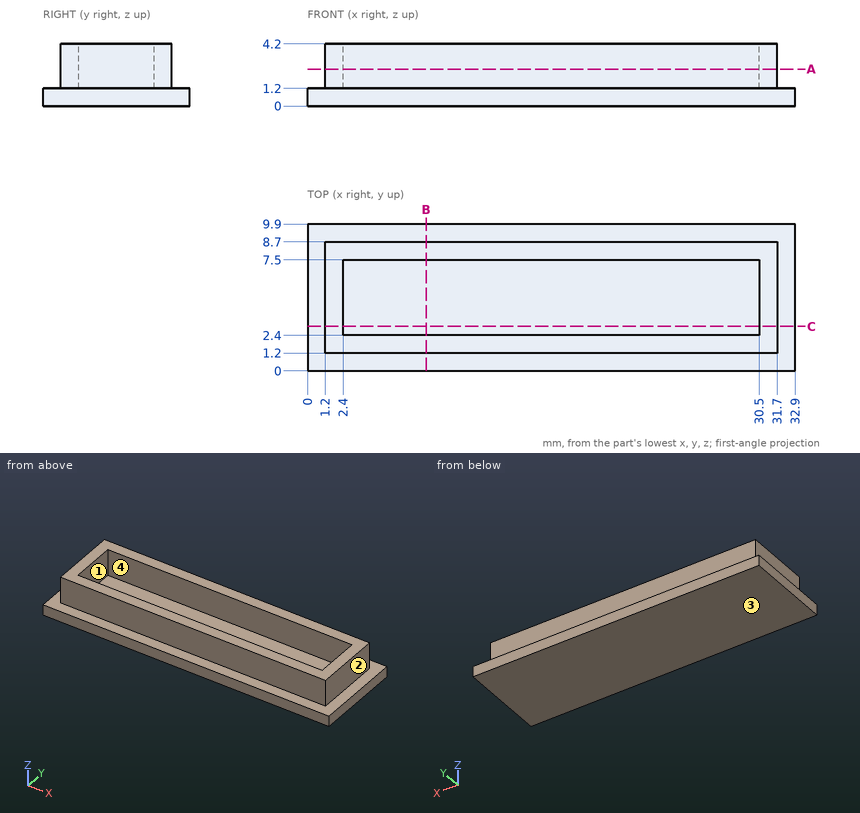
Geometry check sheet. Reference: drawing and pictorial views, mm from the part's lowest x, y, z. Coordinates: 2 decimals unless noted, no trailing zeros. Write each loop counter-clockwise with the first axis right and the second up, starting at its lowest first coordinate (ties: lowest second). Pieces come first, ordered by that corner, then holes.
Item 1: Cross-section at A-A on z = 2.5. Record the boundary of the cut face in (x, y).
Numbers:
outline: (1.2, 1.2) - (31.7, 1.2) - (31.7, 8.7) - (1.2, 8.7) - close; hole (2.4, 2.4) - (30.5, 2.4) - (30.5, 7.5) - (2.4, 7.5) - close
Item 2: Cross-section at C-C on y = 3. Record the boundary of the cut face in (x, z), then the cut area to 3 significant figures.
Numbers:
outline: (0, 0) - (32.9, 0) - (32.9, 1.2) - (31.7, 1.2) - (31.7, 4.2) - (30.5, 4.2) - (30.5, 1.2) - (2.4, 1.2) - (2.4, 4.2) - (1.2, 4.2) - (1.2, 1.2) - (0, 1.2) - close
area: 46.7 mm2
Item 3: Depth check by flat-ended pin: pin 1 Ø2.5 at (x, z) = (14.5, 3) entering from +Y; pin 2 Ø2.5 at (x, y) = (19, 6) entering from +Z; pin 3 Ø0.9 at (y, z) = (4, 3.5) entering from -X. Enter the tip coordinate at first touch or a pass-through.
Numbers:
pin 1: stops at y = 8.7
pin 2: stops at z = 1.2
pin 3: stops at x = 1.2
Item 4: Cross-section at B-B on x = 8. Record the boundary of the cut face in (y, z), then the cut area to 3 significant figures.
Numbers:
outline: (0, 0) - (9.9, 0) - (9.9, 1.2) - (8.7, 1.2) - (8.7, 4.2) - (7.5, 4.2) - (7.5, 1.2) - (2.4, 1.2) - (2.4, 4.2) - (1.2, 4.2) - (1.2, 1.2) - (0, 1.2) - close
area: 19.1 mm2
Item 5: Mould release check, pull along X, two halves, no side actions. Record for the marked faces 1, 2, 3 and 4: released by +X, released by -X, zero draft, split by the parting line, or undercut.
Numbers:
face 1: undercut
face 2: released by +X
face 3: zero draft
face 4: undercut
Item 6: Scan lines: probe 1 along Y at (x, z) = (27, 1.5); probe 2 along X at (y, z) = (4.5, 3.45); probe 3 along Z at (x, y) = (26, 4). Record each from-to range of solid material in increasing order.
Numbers:
probe 1: y = 1.2 to 2.4, 7.5 to 8.7
probe 2: x = 1.2 to 2.4, 30.5 to 31.7
probe 3: z = 0 to 1.2
